The model under review builds one solid part; all positions refer to its coordinate system, in mm. A direction names the side the tool comes from. Round coordinates to 2 decimals unless told otherwise and drop trailing zeros. Order: outer loops, then holes, each group sorted by start corner. A loop starts at its lowest first (then second) coordinate and runs counter-clockwise, first axis right, second up. Notation, with made-up numbers: M 51.5,-6.5 L 58.5,-6.5 A33 ccw 58.5,24.5 Z; hole C 64.25,62 d7. An arc over 180 degrees is marked long. Answer as a JSON object with one key per item and string values. Group by question number.
1) Consider section A-A, the plane y = 6. Write out the cut boundary in (x, z), then the cut area to 3 significant figures.
2) Insertion check: pin 1 Ø1 at (x, z) = (-16, 9.5) entering from +Y; pin 2 Ø6.5 at (x, z) = (-13.5, 5.5) entering from -Y; pin 3 Ø1.5 at (y, z) = (30, 9) entering from -X. Each pin has a flat end and moves straight along its axis. Give the tip position at first contact, or say it passes through.
3) Consider section D-D, the plane z = 2.5. Write out the cut boundary in (x, y), then the cut area to 3 significant figures.
4) For faces 1 (the flat face through (-24, 0, 6)), 2 (the flat face through (-5, 13, 6)), list the 3-axis set-ups (+Z, -Z, +X, -X, +Y, -Y) from which the entire face can be reached by the end or side of a thin tool; tool diameter is ignored.
5) Consider section C-C, the plane y = 25. Write out the cut boundary in (x, z).
6) Consider section B-B, the plane z = 6.35. Write out the cut boundary in (x, y), then the cut area to 3 significant figures.
7) To check wall thickness, follow line 1 (X direction, y = 17, z = 2.25); line 2 (Y direction, x = -3.2, z = 6.35); line 3 (Y direction, x = -22, z = 7.5). State the ranges of each line that lie inside material, in increasing order.
8) The part is to be moulded in two halves that separate along Y. For faces 3 (the flat face through (-13, 26.2, 6)), 4 (the flat face through (-26, 13, 6)), 5 (the cylindrical face through (-2.465, 4.053, 8.889)), say which applies: +Y half, -Y half, draft (parallel to the pull), parting line (faces both ways), or undercut.
```python
from build123d import *

# Parameters (mm, degrees)
BOSS_EXTRUDE1_DEPTH = 12.7
SKETCH2_R           = 3.2
CUT_EXTRUDE1_DEPTH  = 27


with BuildPart() as part:
    # Sketch1 → Boss-Extrude1 (new body)
    with BuildSketch(Plane.XY):
        with BuildLine():
            Line((0, 0), (0, 26.2))
            ThreePointArc((0, 26.2), (-13, 33.716685226), (-26, 26.2))
            Line((-26, 26.2), (-26, 0))
            Line((-26, 0), (-21, 0))
            Line((-21, 0), (-21, 26.2))
            Line((-21, 26.2), (-5, 26.2))
            Line((-5, 26.2), (-5, 0))
            Line((-5, 0), (0, 0))
        make_face()
    extrude(amount=BOSS_EXTRUDE1_DEPTH)

    # Sketch2 → Cut-Extrude1 (cut, through all)
    with BuildSketch(Plane(origin=(0, 0, 0), x_dir=(0, 0, -1), z_dir=(1, 0, 0))):
        with Locations((-6.35, 6)):
            Circle(SKETCH2_R)
    extrude(amount=-CUT_EXTRUDE1_DEPTH, mode=Mode.SUBTRACT)


solid = part.part
```
Results list:
{
 "1": {"outline": "M -26,0 L -21,0 L -21,3.15 L -26,3.15 Z; M -26,9.55 L -21,9.55 L -21,12.7 L -26,12.7 Z; M -5,0 L 0,0 L 0,3.15 L -5,3.15 Z; M -5,9.55 L 0,9.55 L 0,12.7 L -5,12.7 Z", "area": "63.0 mm^2"},
 "2": {"pin 1": "y = 33.51", "pin 2": "y = 26.2", "pin 3": "x = -23.68"},
 "3": {"outline": "M -26,0 L -21,0 L -21,26.2 L -5,26.2 L -5,0 L 0,0 L 0,26.2 A15 ccw -26,26.2 Z", "area": "401 mm^2"},
 "4": {"face 1": "+Z, -Z, +X, -X, -Y", "face 2": "+Z, -Z, -Y"},
 "5": {"outline": "M -26,0 L -21,0 L -21,12.7 L -26,12.7 Z; M -5,0 L 0,0 L 0,12.7 L -5,12.7 Z"},
 "6": {"outline": "M -26,0 L -21,0 L -21,2.8 L -26,2.8 Z; M -26,9.2 L -21,9.2 L -21,26.2 L -5,26.2 L -5,9.2 L 0,9.2 L 0,26.2 A15 ccw -26,26.2 Z; M -5,0 L 0,0 L 0,2.8 L -5,2.8 Z", "area": "337 mm^2"},
 "7": {"line 1": "-26 to -21, -5 to 0", "line 2": "0 to 2.8, 9.2 to 30.07", "line 3": "0 to 3.01, 8.99 to 30.72"},
 "8": {"face 3": "-Y half", "face 4": "draft", "face 5": "undercut"}
}
